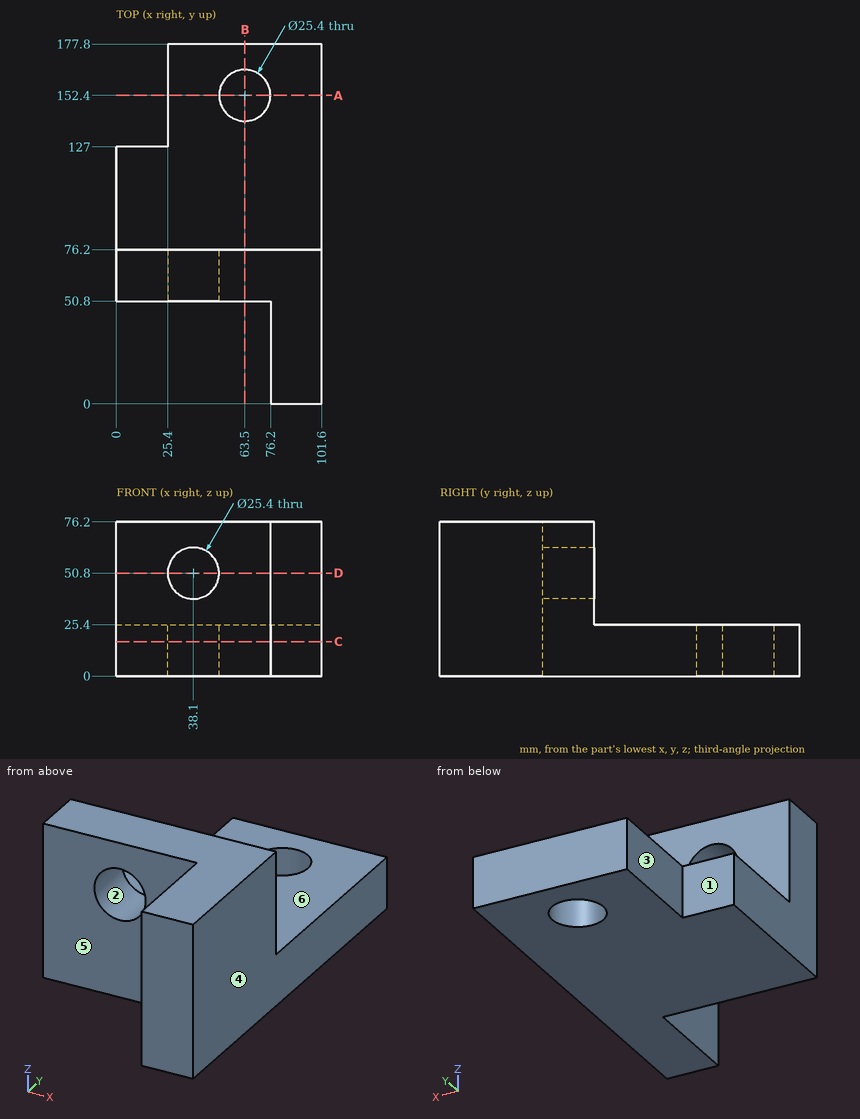
Geometry check sheet. Reference: drawing and pictorial views, mm from the part's lowest x, y, z. A direction names the side the tool comes from. Give positions to 0.01 mm unless a question says otherwise; leave off trailing zeros. Order: outer loops, then holes, each group sorted by start corner. A loop starts at its lowest first (then second) coordinate and runs counter-clockwise, first axis right, second up. Notation, with made-up numbers: M 55.5,9 L 89.5,9 A22 ccw 89.5,34 Z; hole C 63,-3 d10. An arc over 180 degrees is marked long. Answer in a Markdown table with one row per item.
1) Thickness scan on L1, parallel to Z at x = 38.1, y = 56.75; L2, parallel to Y at x = 63, z = 13; L3, parallel to Y at x = 48, z = 18. Record the ranges inside material, lowest first. Write a range as [from, to].
Filled sheet:
| item | result |
|---|---|
| L1 | z = [0, 38.1], [63.5, 76.2] |
| L2 | y = [50.8, 139.71], [165.09, 177.8] |
| L3 | y = [50.8, 177.8] |
2) Cross-section at D-D, the plane z = 50.8. Enter the section's corners in (x, y), plus the area to 3 significant figures.
Filled sheet:
| item | result |
|---|---|
| outline | M 0,50.8 L 25.4,50.8 L 25.4,76.2 L 0,76.2 Z; M 50.8,50.8 L 76.2,50.8 L 76.2,0 L 101.6,0 L 101.6,76.2 L 50.8,76.2 Z |
| area | 3,230 mm2 |
3) Gauge pin test, flat ends, axial feed: P1, Ø10, axis at x = 28, y = 76, coming from the -Z side; P2, Ø8, axis at x = 32.5, z = 40, coming from the -Y side; P3, Ø20.5, axis at y = 143, z = 8, coming from the -X side; P4, Ø12, axis at x = 42.5, y = 83, coming from the +Z side. Record the tip position at first contact, or that the pin passes through.
Filled sheet:
| item | result |
|---|---|
| P1 | stops at z = 0 |
| P2 | stops at y = 50.8 |
| P3 | stops at x = 25.4 |
| P4 | stops at z = 25.4 |
4) Cross-section at B-B, the plane x = 63.5. Enter the section's corners in (y, z), plus the area to 3 significant figures.
Filled sheet:
| item | result |
|---|---|
| outline | M 50.8,0 L 139.7,0 L 139.7,25.4 L 76.2,25.4 L 76.2,76.2 L 50.8,76.2 Z; M 165.1,0 L 177.8,0 L 177.8,25.4 L 165.1,25.4 Z |
| area | 3,870 mm2 |
5) Access from +Z, -Z, +X, -X, +Y, -Y to the whole of each face (thin tool, end or side, straight path). Record for the marked faces 4, 5 and 6.
Filled sheet:
| item | result |
|---|---|
| face 4 | +Z, -Z, +X, +Y, -Y |
| face 5 | +Z, -Z, -X, -Y |
| face 6 | +Z, +X, -X, +Y |
6) Cross-section at A-A, the plane y = 152.4. Enter the section's corners in (x, z).
Filled sheet:
| item | result |
|---|---|
| outline | M 25.4,0 L 50.8,0 L 50.8,25.4 L 25.4,25.4 Z; M 76.2,0 L 101.6,0 L 101.6,25.4 L 76.2,25.4 Z |
7) Release check for a two-part mould opening along X. For the marked faces 1, 2 and 3 record: +X half, -X half, draft (parallel to the pull), parting line (faces both ways), or undercut.
Filled sheet:
| item | result |
|---|---|
| face 1 | draft |
| face 2 | undercut |
| face 3 | -X half |
8) Cross-section at C-C, the plane z = 17. Enter the section's corners in (x, y), plus the area to 3 significant figures.
Filled sheet:
| item | result |
|---|---|
| outline | M 0,50.8 L 76.2,50.8 L 76.2,0 L 101.6,0 L 101.6,177.8 L 25.4,177.8 L 25.4,127 L 0,127 Z; hole C 63.5,152.4 d25.4 |
| area | 12,400 mm2 |
